Part print with two shaded views. Sizes in mm from the minimum x, y, z corner. Coordinates: 2 decimals unless noted, no trailing zeros. Order: outer loops, then holes, each group sorted by start corner. A loop starts at its lowest first (then second) coordinate and runs counter-clockwise, first axis right, second up. Notation, with made-up numbers: (1, 63) - (53, 63) arc R3 cw to (53, 68) - close; hole circle Ø6 at (83, 54). An arc over 180 degrees is marked (long way). Return JSON: item names as keys, results as strings.
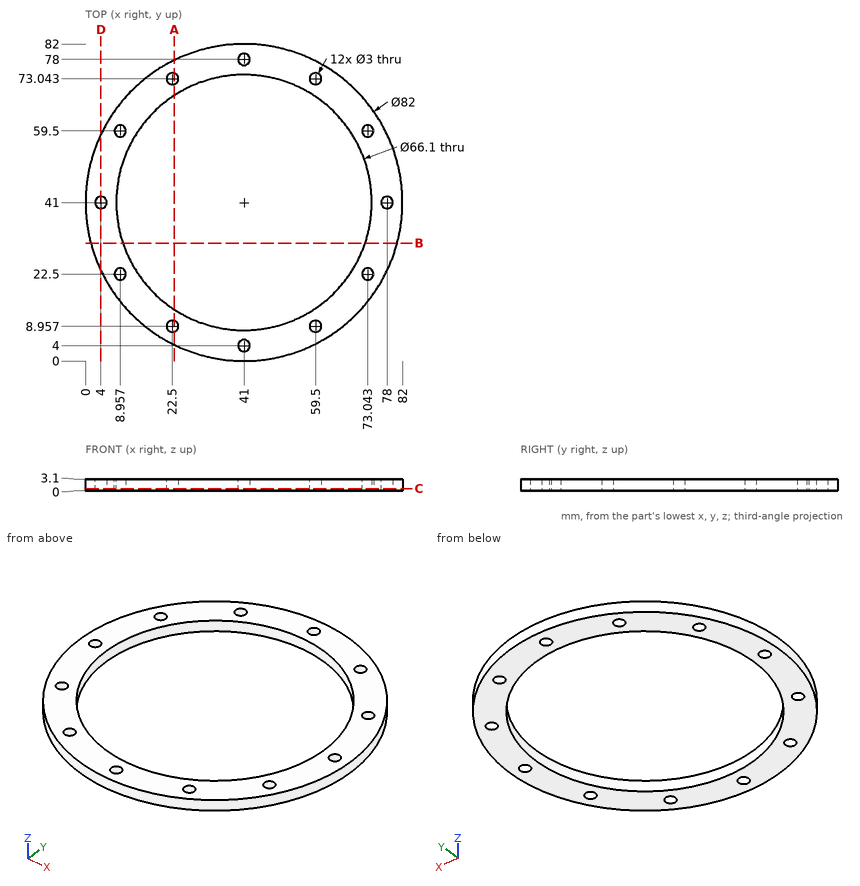
Item 1: Drop a flat-ended pin along its axis: P1, Ø1.5, axis at y = 17, z = 1.5, coming from the -X side. Give the stop position or say it passes through.
Findings below:
{"P1": "stops at x = 7.23"}
Item 2: Band-saw the part on C-C, the plane z = 0.6. Count the separate pieces of the cut face and the enclosed holes in it, then the cut area to 3 significant figures.
Findings below:
{"separate pieces": "1", "enclosed holes": "13", "area": "1,760 mm²"}
Item 3: Band-saw the part on D-D, the plane x = 4. List the corners of the cut face in (y, z), then the cut area to 3 significant figures.
Findings below:
{"outline": "(23.34, 0) - (39.5, 0) - (39.5, 3.1) - (23.34, 3.1) - close; (42.5, 0) - (58.66, 0) - (58.66, 3.1) - (42.5, 3.1) - close", "area": "100 mm²"}
Item 4: Band-saw the part on B-B, the plane y = 30.5. List the corners of the cut face in (x, z).
Findings below:
{"outline": "(1.37, 0) - (9.66, 0) - (9.66, 3.1) - (1.37, 3.1) - close; (72.34, 0) - (80.63, 0) - (80.63, 3.1) - (72.34, 3.1) - close"}
Item 5: Wall check: L1, parallel to Y at x = 41, z = 2.35; L2, parallel to X at y = 21.5, z = 0.5 (1 decimal); L3, parallel to X at y = 59.5, z = 1. Give the ranges that are in metal, low to high. Write a range as [from, to].
Findings below:
{"L1": "y = [0, 2.5], [5.5, 7.95], [74.05, 76.5], [79.5, 82]", "L2": "x = [4.9, 7.8], [10.1, 14.3], [67.7, 71.9], [74.2, 77.1]", "L3": "x = [4.41, 7.46], [10.46, 13.61], [68.39, 71.54], [74.54, 77.59]"}
Item 6: Band-saw the part on A-A, the plane x = 23. List the corners of the cut face in (y, z), then the cut area to 3 significant figures.
Findings below:
{"outline": "(4.16, 0) - (7.54, 0) - (7.54, 3.1) - (4.16, 3.1) - close; (10.37, 0) - (13.28, 0) - (13.28, 3.1) - (10.37, 3.1) - close; (68.72, 0) - (71.63, 0) - (71.63, 3.1) - (68.72, 3.1) - close; (74.46, 0) - (77.84, 0) - (77.84, 3.1) - (74.46, 3.1) - close", "area": "39.0 mm²"}
